CAD build for the part. Positions are in the model's coordinates, mm. A direction names the side the tool comes from. Give positions to 0.01 mm unless a question says otherwise; leave off trailing zeros. Write each loop counter-clockwise with the first axis right and the second up, starting at its lowest first coordinate (ties: lowest second). Pieces come first, ordered by that corner, then holes. Notation, with made-up numbers: (82, 38) -> (104, 38) arc R33 cw to (104, 77) -> close; hole circle Ø8 at (21.5, 54.25). An arc over 180 degrees is marked (long way). Answer as a JSON object with one key per item and string values.
```python
from build123d import *

# Parameters (mm, degrees)
F1_DEPTH = 76.2


with BuildPart() as f1:
    # F0 (on Front) → F1 (new body)
    with BuildSketch(Plane.XZ):
        with BuildLine():
            Line((231.2415951175, 231.2415951175), (327.025, 0))
            ThreePointArc((327.025, 0), (302.1317041195, 125.1470494692), (231.2415951175, 231.2415951175))
        make_face()
        Polygon((0, 0), (327.025, 0), (231.2415951175, 231.2415951175), align=None)
        with BuildLine():
            ThreePointArc((231.2415951175, -231.2415951175), (302.1317041195, -125.1470494692), (327.025, 0))
            Line((327.025, 0), (231.2415951175, -231.2415951175))
        make_face()
        Polygon((231.2415951175, -231.2415951175), (327.025, 0), (0, 0), align=None)
        with BuildLine():
            Line((0, 327.025), (231.2415951175, 231.2415951175))
            ThreePointArc((231.2415951175, 231.2415951175), (125.1470494692, 302.1317041195), (0, 327.025))
        make_face()
        Polygon((0, 0), (231.2415951175, 231.2415951175), (0, 327.025), align=None)
        with BuildLine():
            ThreePointArc((0, -327.025), (125.1470494692, -302.1317041195), (231.2415951175, -231.2415951175))
            Line((231.2415951175, -231.2415951175), (0, -327.025))
        make_face()
        Polygon((0, -327.025), (231.2415951175, -231.2415951175), (0, 0), align=None)
        Polygon((0, -327.025), (0, 0), (-231.2415951175, -231.2415951175), align=None)
        Polygon((-231.2415951175, 231.2415951175), (0, 0), (0, 327.025), align=None)
        Polygon((-327.025, 0), (0, 0), (-231.2415951175, 231.2415951175), align=None)
        Polygon((-231.2415951175, -231.2415951175), (0, 0), (-327.025, 0), align=None)
        with BuildLine():
            Line((-231.2415951175, 231.2415951175), (0, 327.025))
            ThreePointArc((0, 327.025), (-125.1470494692, 302.1317041195), (-231.2415951175, 231.2415951175))
        make_face()
        with BuildLine():
            Line((0, -409.5032856623), (0, -327.025))
            ThreePointArc((0, -327.025), (-125.1470494692, -302.1317041195), (-231.2415951175, -231.2415951175))
            Line((-231.2415951175, -231.2415951175), (-289.56255021, -289.56255021))
            Line((-289.56255021, -289.56255021), (0, -409.5032856623))
        make_face()
        with BuildLine():
            ThreePointArc((-231.2415951175, -231.2415951175), (-125.1470494692, -302.1317041195), (0, -327.025))
            Line((0, -327.025), (-231.2415951175, -231.2415951175))
        make_face()
        with BuildLine():
            ThreePointArc((-327.025, 0), (-302.1317041195, -125.1470494692), (-231.2415951175, -231.2415951175))
            Line((-231.2415951175, -231.2415951175), (-327.025, 0))
        make_face()
        with BuildLine():
            Line((-327.025, 0), (-231.2415951175, 231.2415951175))
            ThreePointArc((-231.2415951175, 231.2415951175), (-302.1317041195, 125.1470494692), (-327.025, 0))
        make_face()
    extrude(amount=F1_DEPTH)


solid = f1.part
```
1) Wall check: probe 1 along Z at (x, y) = (-237, -14.5); probe 2 along Z at (x, y) = (12, -52.5); probe 3 along Z at (x, y) = (49, -22). Give the ranges that are in metal, low to high.
Model answer:
{"probe 1": "z = -311.33 to -237, -225.34 to 225.34", "probe 2": "z = -326.8 to 326.8", "probe 3": "z = -323.33 to 323.33"}
2) Slice it at A-A (y = -34.5). List the corners of the cut face in (x, z) (3 decimals).
Model answer:
{"outline": "(-289.563, -289.563) -> (0, -409.503) -> (0, -327.025) arc R327.025 ccw (long way) to (-231.242, -231.242) -> close"}
3) Pin check, flat tips, straight feed: pin 1 (6 mm diameter, centred on y = -68, z = -288.5, fed in from -X); pin 2 (23 mm diameter, centred on y = -31.5, z = -387, fed in from +X); pin 3 (4 mm diameter, centred on y = -44.5, z = 141.5, fed in from +X). Stop position of each tip, or through.
Model answer:
{"pin 1": "stops at x = -289.56", "pin 2": "stops at x = 0", "pin 3": "stops at x = 295.78"}
4) 3-axis set-ups, long thin cutter, end or side, ignore diameter. For faces 1 (the flat face through (0, -38, -369)), 2 (the flat face through (-5, -76.2, -36)), 3 (the flat face through (-260, -38, -260)): which of +Z, -Z, +X, -X, +Y, -Y reach the whole face in a straight line?
Model answer:
{"face 1": "-Z, +X, +Y, -Y", "face 2": "+Z, -Z, +X, -X, -Y", "face 3": "-X, +Y, -Y"}
5) Slice it at B-B (x = 43). List the corners of the cut face in (y, z), then the cut area to 3 significant figures.
Model answer:
{"outline": "(-76.2, -324.19) -> (0, -324.19) -> (0, 324.19) -> (-76.2, 324.19) -> close", "area": "49,400 mm2"}
6) Slice it at C-C (z = -165). List the corners of the cut face in (x, y), then the cut area to 3 significant figures.
Model answer:
{"outline": "(-282.35, -76.2) -> (282.35, -76.2) -> (282.35, 0) -> (-282.35, 0) -> close", "area": "43,000 mm2"}
